```python
from build123d import *

# Parameters (mm, degrees)
SKETCH1_W           = 609.6
SKETCH1_H           = 50.8
BOSS_EXTRUDE1_DEPTH = 25.4
FILLET1_R           = 12.7
SKETCH4_R           = 19.05
CUT_EXTRUDE1_DEPTH  = 613.240116294
SKETCH5_R           = 19.05
CUT_EXTRUDE2_DEPTH  = 613.240116294
SKETCH2_R           = 19.05
CUT_EXTRUDE3_DEPTH  = 613.240116294


with BuildPart() as part:
    # Sketch1 → Boss-Extrude1 (new body)
    with BuildSketch(Plane.XY):
        with Locations((304.8, 25.4)):
            Rectangle(SKETCH1_W, SKETCH1_H)
    extrude(amount=BOSS_EXTRUDE1_DEPTH)

    # Fillet1
    fillet1_edges = [part.edges().sort_by_distance(p)[0] for p in [
        (0, 50.8, 12.7),
        (609.6, 50.8, 12.7),
        (609.6, 0, 12.7),
        (0, 0, 12.7),
    ]]
    fillet(fillet1_edges, radius=FILLET1_R)

    # Sketch4 → Cut-Extrude1 (cut, through all)
    with BuildSketch(Plane.XY.offset(25.4)):
        with Locations((584.2, 25.4)):
            Circle(SKETCH4_R)
    extrude(amount=-CUT_EXTRUDE1_DEPTH, mode=Mode.SUBTRACT)

    # Sketch5 → Cut-Extrude2 (cut, through all)
    with BuildSketch(Plane(origin=(0, 0, 0), x_dir=(-1, 0, 0), z_dir=(0, 0, -1))):
        with Locations((-304.8, 25.4)):
            Circle(SKETCH5_R)
    extrude(amount=-CUT_EXTRUDE2_DEPTH, mode=Mode.SUBTRACT)

    # Sketch2 → Cut-Extrude3 (cut, through all)
    with BuildSketch(Plane.XY.offset(25.4)):
        with Locations((25.4, 25.4)):
            Circle(SKETCH2_R)
    extrude(amount=-CUT_EXTRUDE3_DEPTH, mode=Mode.SUBTRACT)


solid = part.part
```
Geometry check sheet. Reference: the model listing, model coordinates, mm. Give positions to 0.01 mm unless a question says otherwise; leave off trailing zeros. Order: outer loops, then holes, each group sorted by start corner. A loop starts at its lowest first (then second) coordinate and runs counter-clockwise, first axis right, second up. Notation, with made-up numbers: (4.5, 77) - (37.5, 77) arc R18 cw to (37.5, 86) - close; hole circle Ø3 at (-0.5, -16). An arc over 180 degrees is marked (long way). Write item = value, one per line. Start each with the question number.
1) Section check C-C (x = 25.4). Enter the section's corners in (y, z), then the cut area to 3 significant figures.
2) Section check B-B (z = 7.25). Enter the section's corners in (x, y), then the cut area to 3 significant figures.
3) Scan lines: L1, parallel to X at y = 26, z = 21.75; L2, parallel to Y at x = 25.4, z = 7.5; L3, parallel to X at y = 20.5, z = 17.25. Record each from-to range of solid material in increasing order.
4) Draft check along Y on faces 1 (the flat face through (301, 0, 13)), 2 (the cylindrical face through (605.98, 46.98, 12.88)), 3 (the cylindrical face through (601.797, 18.104, 12.878)). Enter one of: released by +Y, released by -Y, zero draft, split by the parting line, or undercut.
5) Section check D-D (x = 314.5). Enter the section's corners in (y, z), then the cut area to 3 significant figures.
6) Section check A-A (y = 25.4). Enter the section's corners in (x, z), then the cut area to 3 significant figures.
7) Gauge pin test, flat end, axial feed: pin 1 Ø5 at (y, z) = (39, 4) entering from -X. Record the tip position at first contact, or that the pin passes through.
Geometry check:
q1.outline = (0, 0) - (6.35, 0) - (6.35, 25.4) - (0, 25.4) - close; (44.45, 0) - (50.8, 0) - (50.8, 25.4) - (44.45, 25.4) - close
q1.area = 323 mm2
q2.outline = (0, 12.7) arc R12.7 ccw to (12.7, 0) - (596.9, 0) arc R12.7 ccw to (609.6, 12.7) - (609.6, 38.1) arc R12.7 ccw to (596.9, 50.8) - (12.7, 50.8) arc R12.7 ccw to (0, 38.1) - close; hole circle Ø38.1 at (25.4, 25.4); hole circle Ø38.1 at (304.8, 25.4); hole circle Ø38.1 at (584.2, 25.4)
q2.area = 27,400 mm2
q3.L1 = 0 to 6.36, 44.44 to 285.76, 323.84 to 565.16, 603.24 to 609.6
q3.L2 = 0 to 6.35, 44.45 to 50.8
q3.L3 = 0 to 6.99, 43.81 to 286.39, 323.21 to 565.79, 602.61 to 609.6
q4.face_1 = released by -Y
q4.face_2 = released by +Y
q4.face_3 = undercut
q5.outline = (0, 0) - (9, 0) - (9, 25.4) - (0, 25.4) - close; (41.8, 0) - (50.8, 0) - (50.8, 25.4) - (41.8, 25.4) - close
q5.area = 457 mm2
q6.outline = (0, 0) - (6.35, 0) - (6.35, 25.4) - (0, 25.4) - close; (44.45, 0) - (285.75, 0) - (285.75, 25.4) - (44.45, 25.4) - close; (323.85, 0) - (565.15, 0) - (565.15, 25.4) - (323.85, 25.4) - close; (603.25, 0) - (609.6, 0) - (609.6, 25.4) - (603.25, 25.4) - close
q6.area = 12,600 mm2
q7.pin_1 = 0
